Here's how the part is built. I have some questions about the finished solid (model axes, mm). A direction names the side the tool comes from. Give positions to 0.01 mm unless a question says otherwise; leave off trailing zeros. Order: outer loops, then holes, each group sorted by start corner. A loop starts at its lowest first (then second) coordinate and runs counter-clockwise, first axis right, second up. Notation, with made-up numbers: M 5.5,28.5 L 18.5,28.5 A23 ccw 18.5,67.5 Z; hole C 40,-2.75 d11. An arc over 180 degrees is marked long. Use CSV: the item, a comma, the result in double quotes. Start each with the question number.
```python
from build123d import *

# Parameters (mm, degrees)
SKETCH1_R           = 3.429
SKETCH1_W           = 27.94
SKETCH1_H           = 8.89
BOSS_EXTRUDE1_DEPTH = 6.35


with BuildPart() as part:
    # Sketch1 → Boss-Extrude1 (new body)
    with BuildSketch(Plane(origin=(0, 0, 0), x_dir=(1, 0, 0), z_dir=(0, 1, 0))):
        with BuildLine():
            Line((13.870085237, 15.767711804), (16.343875029, 16.343875029))
            Line((16.343875029, 16.343875029), (15.767711804, 13.870085237))
            ThreePointArc((15.767711804, 13.870085237), (21, 0), (15.767711804, -13.870085237))
            Line((15.767711804, -13.870085237), (16.343875029, -16.343875029))
            Line((16.343875029, -16.343875029), (13.870085237, -15.767711804))
            ThreePointArc((13.870085237, -15.767711804), (0, -21), (-13.870085237, -15.767711804))
            Line((-13.870085237, -15.767711804), (-16.343875029, -16.343875029))
            Line((-16.343875029, -16.343875029), (-15.767711804, -13.870085237))
            ThreePointArc((-15.767711804, -13.870085237), (-21, 0), (-15.767711804, 13.870085237))
            Line((-15.767711804, 13.870085237), (-16.343875029, 16.343875029))
            Line((-16.343875029, 16.343875029), (-13.870085237, 15.767711804))
            ThreePointArc((-13.870085237, 15.767711804), (0, 21), (13.870085237, 15.767711804))
        make_face()
        with Locations(Location((-8.382, 8.382, 0), (0, 0, 270))):
            Circle(SKETCH1_R, mode=Mode.SUBTRACT)
        with Locations(Location((8.382, 8.382, 0), (0, 0, 270))):
            Circle(SKETCH1_R, mode=Mode.SUBTRACT)
        with Locations((0, -7.62)):
            Rectangle(SKETCH1_W, SKETCH1_H, mode=Mode.SUBTRACT)
    extrude(amount=BOSS_EXTRUDE1_DEPTH)


solid = part.part
```
Q1. For faces 5 (the face through (0, 3, 12.065)), 6 (the face through (-15.12, 3.13, -16.06)), 7 (the face through (15.12, 3.13, 16.06)), which set-ups out of +Z, -Z, +X, -X, +Y, -Y let a thin tool reach every point of the face, with its end or its side?
Q2. For P1, Ø3, axis at y = 4.5, z = 9.5, coming from the +X side; P2, Ø1, axis at y = 2.5, z = -2, coming from the -X side; P3, Ø5.5, axis at x = 8.382, z = -8.382, coming from the +Y side; P4, Ø11, axis at x = -8.382, z = -8.382, coming from the +Y side, each with a flat end and sliding along its axis, tell me the tip position at first contact or that it passes through.
Q3. I need wall thicknesses on line 1 (X direction, y = 5, z = -10.5); line 2 (Z direction, x = 7.5, y = 1.5) (3 decimals); line 3 (Z direction, x = -10, y = 6.25) (3 decimals). Which ranges of each line are inside material? Lowest first, please. Write a range as [from, to].
Q4. We'd pull the mould along Z, two halves only. Please class faces 1 (the face through (0, 0, 0)), 2 (the face through (13.97, 3, 8)), 3 (the face through (-15.09, 3.13, 16.05)), 4 (the face through (15.09, 3.13, -16.05)): pulls with the +Z half, pulls with the -Z half, needs draft (parallel to the pull), parting line crosses it, or undercut.
Q5. Imagine slicing it at D-D, the plane z = 6.5. Please give me the cut outline in (x, y), then the cut area to 3 significant figures.
Q6. Imagine slicing it at C-C, the plane y = 0.5. Please give me the cut outline in (x, z) (3 decimals).
Q7. Imagine slicing it at A-A, the plane x = -7. Please give me the cut outline in (y, z) (3 decimals), then the cut area to 3 significant figures.
Q8. Imagine slicing it at B-B, the plane z = -7.5. Please give me the cut outline in (x, y).
Reply:
1,face 5,"+Y, -Y"
1,face 6,"-Z, +Y, -Y"
1,face 7,"+Z, +Y, -Y"
2,P1,"stops at x = 19.42"
2,P2,"stops at x = -20.95"
2,P3,"passes through"
2,P4,"stops at y = 6.35"
3,line 1,"x = [-18.19, -11.08], [-5.69, 5.69], [11.08, 18.19]"
3,line 2,"z = [-19.615, -11.696], [-5.068, 3.175], [12.065, 19.615]"
3,line 3,"z = [-18.466, -11.405], [-5.359, 3.175], [12.065, 18.466]"
4,face 1,"needs draft"
4,face 2,"undercut"
4,face 3,"pulls with the +Z half"
4,face 4,"pulls with the -Z half"
5,outline,"M -19.97,0 L -13.97,0 L -13.97,6.35 L -19.97,6.35 Z; M 13.97,0 L 19.97,0 L 19.97,6.35 L 13.97,6.35 Z"
5,area,"76.2 mm^2"
6,outline,"M -16.344,-16.344 L -13.87,-15.768 A21 ccw 13.87,-15.768 L 16.344,-16.344 L 15.768,-13.87 A21 ccw 15.768,13.87 L 16.344,16.344 L 13.87,15.768 A21 ccw -13.87,15.768 L -16.344,16.344 L -15.768,13.87 A21 ccw -15.768,-13.87 Z; hole M -13.97,3.175 L 13.97,3.175 L 13.97,12.065 L -13.97,12.065 Z; hole C -8.382,-8.382 d6.858; hole C 8.382,-8.382 d6.858"
7,outline,"M 0,-19.799 L 6.35,-19.799 L 6.35,-11.52 L 0,-11.52 Z; M 0,-5.244 L 6.35,-5.244 L 6.35,3.175 L 0,3.175 Z; M 0,12.065 L 6.35,12.065 L 6.35,19.799 L 0,19.799 Z"
7,area,"155 mm^2"
8,outline,"M -19.62,0 L -11.7,0 L -11.7,6.35 L -19.62,6.35 Z; M -5.07,0 L 5.07,0 L 5.07,6.35 L -5.07,6.35 Z; M 11.7,0 L 19.62,0 L 19.62,6.35 L 11.7,6.35 Z"
